Could you check a few things on this model? Use its own coordinates, in mm. A direction names the side the tool comes from. Coordinates: 2 decimals unless noted, no trailing zeros. Loops run counter-clockwise (first coordinate to the right, second up) from the corner with the lowest first, then second, coordinate; pieces in that order, holes last.
from build123d import *

# Parameters (mm, degrees)
SKETCH1_R           = 1.25
BOSS_EXTRUDE1_DEPTH = 3.175
FILLET1_R           = 6.35


with BuildPart() as part:
    # Sketch1 → Boss-Extrude1 (new body)
    with BuildSketch(Plane(origin=(0, 0, 0), x_dir=(1, 0, 0), z_dir=(0, 1, 0))):
        Polygon((15.147658291, 44.238817403), (-25.76324473, 3.302114568), (15.173458104, -37.608788453), (56.084361126, 3.327914382), align=None)
        with Locations(Location((17.840116094, 13.708278644, 0), (0, 0, 270))):
            Circle(SKETCH1_R, mode=Mode.SUBTRACT)
        with Locations(Location((4.768985382, 0.628904831, 0), (0, 0, 270))):
            Circle(SKETCH1_R, mode=Mode.SUBTRACT)
        with Locations(Location((-19.669398793, 3.304035457, 0), (0, 0, 270))):
            Circle(SKETCH1_R, mode=Mode.SUBTRACT)
        with Locations(Location((15.149579179, 38.144971466, 0), (0, 0, 270))):
            Circle(SKETCH1_R, mode=Mode.SUBTRACT)
        with Locations(Location((49.990509247, 3.325999432, 0), (0, 0, 270))):
            Circle(SKETCH1_R, mode=Mode.SUBTRACT)
        with Locations(Location((15.171537216, -31.514942515, 0), (0, 0, 270))):
            Circle(SKETCH1_R, mode=Mode.SUBTRACT)
        Polygon((14.901563134, -5.042362692), (-1.352871962, 11.201828262), (7.263335329, 19.823469227), (23.517770424, 3.579278273), align=None, mode=Mode.SUBTRACT)
    extrude(amount=BOSS_EXTRUDE1_DEPTH)

    # Fillet1
    fillet1_edges = [part.edges().sort_by_distance(p)[0] for p in [
        (-25.76324473, 1.5875, -3.302114568),
        (15.147658291, 1.5875, -44.238817403),
        (56.084361126, 1.5875, -3.327914382),
        (15.173458104, 1.5875, 37.608788453),
    ]]
    fillet(fillet1_edges, radius=FILLET1_R)


solid = part.part
1) For faces 5 (the cylindrical face through (15.08, 1.61, -41.61)), 6 (the flat face through (6.888, 1.565, -2.966)), which set-ups out of +Z, -Z, +X, -X, +Y, -Y let a thin tool reach every point of the face, with its end or its side?
2) Imagine slicing it at D-D on x = 22. List the corners of the cut face in (y, z) for me (3 decimals), plus the area to 3 significant figures.
3) Imagine slicing it at C-C on y = 2.55. List the corners of the cut face in (x, z) for me.
4) Will these pins go through, and if not, where does the flat tip stop? pin 1 (2 mm diameter, centred on x = 17.84, z = -13.71, fed in from -Y); pin 2 (1 mm diameter, centred on x = 19.5, y = 2, fed in from +Z); pin 3 (1.5 mm diameter, centred on x = -3.5, y = 2.5, fed in from -Z).
5) Imagine slicing it at B-B on z = -0.5. List the corners of the cut face in (x, y) for me (3 decimals).
6) If I drill on L1, parallel to Z at x = 5.5, y = 2.6; L2, parallel to Z at x = 5, y = 2.25; L3, parallel to X at y = 1.15, z = -0.5, over which ranges is the centre line in solid material (lowest first)?
7) We'd pull the mould along Z, two halves only. Please class faces 1 (the cylindrical face through (-23.133, 1.61, -3.373)), 2 (the flat face through (-5.084, 1.565, -23.994)), 3 (the cylindrical face through (16.62, 1.57, -13.98)), 4 (the cylindrical face through (-20.89, 1.57, -3.58)): released by +Z, released by -Z, zero draft, split by the parting line, or undercut.
8) Imagine slicing it at A-A on x = 0.5. List the corners of the cut face in (y, z) for me (3 decimals), plus the area to 3 significant figures.
Solved:
1. face 5: -Z, +Y, -Y
1. face 6: +Y, -Y
2. outline: (0, -37.391) - (3.175, -37.391) - (3.175, -5.096) - (0, -5.096) - close; (0, -2.061) - (3.175, -2.061) - (3.175, 30.778) - (0, 30.778) - close
2. area: 207 mm2
3. outline: (-21.27, -7.79) - (10.66, -39.75) arc R6.35 ccw to (19.64, -39.75) - (51.59, -7.82) arc R6.35 ccw to (51.6, 1.16) - (19.66, 33.12) arc R6.35 ccw to (10.68, 33.12) - (-21.27, 1.19) arc R6.35 ccw to start; hole circle Ø2.5 at (-19.67, -3.3); hole (-1.35, -11.2) - (7.26, -19.82) - (23.52, -3.58) - (14.9, 5.04) - close; hole circle Ø2.5 at (4.77, -0.63); hole circle Ø2.5 at (15.15, -38.14); hole circle Ø2.5 at (15.17, 31.51); hole circle Ø2.5 at (17.84, -13.71); hole circle Ø2.5 at (49.99, -3.33)
4. pin 1: passes through
4. pin 2: stops at z = 33.69
4. pin 3: stops at z = -26.33
5. outline: (-22.48, 0) - (3.526, 0) - (3.526, 3.175) - (-22.48, 3.175) - close; (6.012, 0) - (9.356, 0) - (9.356, 3.175) - (6.012, 3.175) - close; (20.44, 0) - (52.791, 0) - (52.791, 3.175) - (20.44, 3.175) - close
6. L1: z = -34.59 to -18.06, -4.35 to -1.64, 0.39 to 27.94
6. L2: z = -34.08 to -17.56, -4.85 to -1.86, 0.6 to 27.44
6. L3: x = -22.48 to 3.53, 6.01 to 9.36, 20.44 to 52.79
7. face 1: split by the parting line
7. face 2: released by -Z
7. face 3: undercut
7. face 4: undercut
8. outline: (0, -29.582) - (3.175, -29.582) - (3.175, -13.056) - (0, -13.056) - close; (0, -9.35) - (3.175, -9.35) - (3.175, 22.945) - (0, 22.945) - close
8. area: 155 mm2
